Verification items for this drawing (mm, ordinates from the low corner). A direction names the side the tool comes from. Coordinates: 2 decimals unless noted, no trailing zeros. Order: outer loops, then holes, each group sorted by start corner. A loop starts at its lowest first (then second) coordinate and runs counter-clockwise, first axis right, second up.
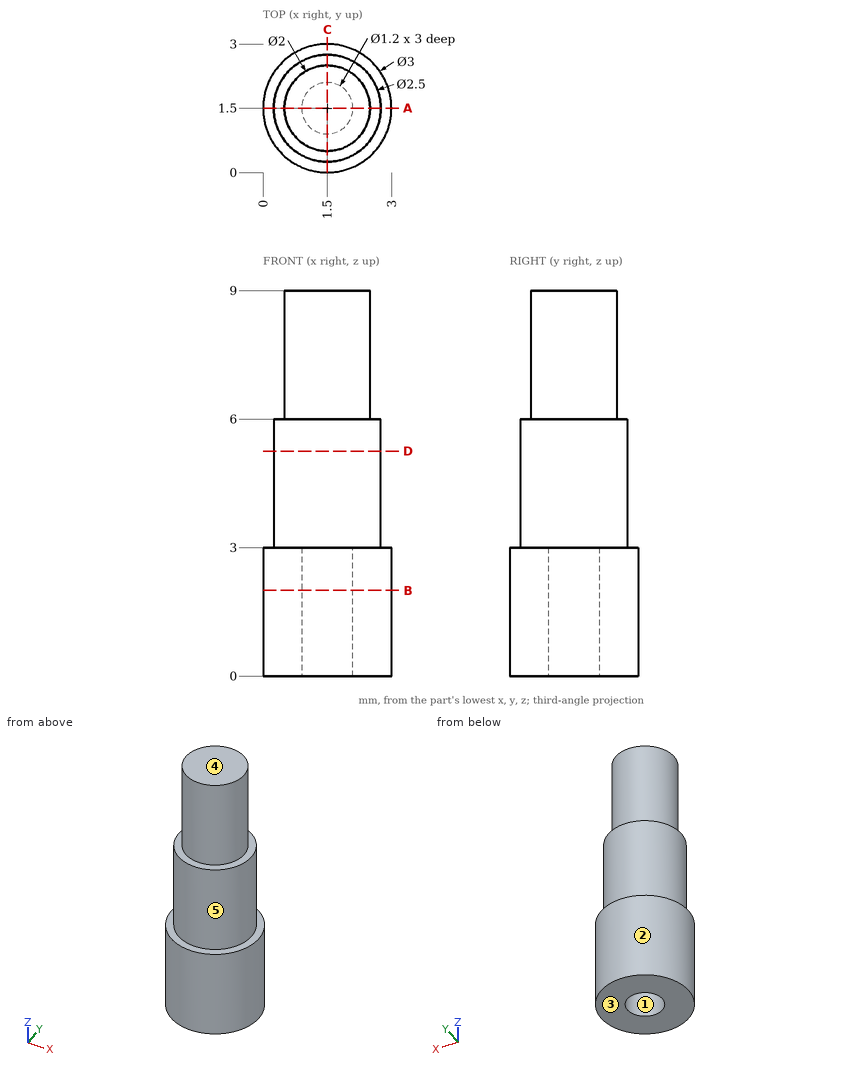
(1) Cross-section at A-A (y = 1.5). Enter the section's corners in (x, z), and give its area (3 significant figures).
Filled in:
outline: (0, 0) - (0.9, 0) - (0.9, 3) - (2.1, 3) - (2.1, 0) - (3, 0) - (3, 3) - (2.75, 3) - (2.75, 6) - (2.5, 6) - (2.5, 9) - (0.5, 9) - (0.5, 6) - (0.25, 6) - (0.25, 3) - (0, 3) - close
area: 18.9 mm2
(2) Cross-section at D-D (z = 5.25). Enter the section's corners in (x, y).
Filled in:
outline: circle Ø2.5 at (1.5, 1.5)
(3) Thickness scan on probe 1 along Y at (x, z) = (1.5, 1.5); probe 2 along Z at (x, y) = (1.65, 1.15); probe 3 along X at (y, z) = (0.75, 3.5). Record the ranges inside material, lowest first.
Filled in:
probe 1: y = 0 to 0.9, 2.1 to 3
probe 2: z = 3 to 9
probe 3: x = 0.5 to 2.5
(4) Release check for a two-part mould opening along Y. For the marked faces 1, 2 and 3 record: +Y half, -Y half, draft (parallel to the pull), parting line (faces both ways), or undercut.
Filled in:
face 1: undercut
face 2: parting line
face 3: draft
(5) Cross-section at B-B (z = 2). Enter the section's corners in (x, y).
Filled in:
outline: circle Ø3 at (1.5, 1.5); hole circle Ø1.2 at (1.5, 1.5)
(6) Go/stop test with a flat-tipped pin: P1, Ø1, axis at x = 1.5, y = 1.5, coming from the -Z side. Record where the tip stops, or that it passes through.
Filled in:
P1: stops at z = 3
(7) Tool access check on the marked faces 4 and 5. Record the directions out of +Z, -Z, +X, -X, +Y, -Y that give a thin tool (end or side, any length) a straight path to the whole face; none if there is none.
Filled in:
face 4: +Z, +X, -X, +Y, -Y
face 5: +Z
